```python
from build123d import *

# Parameters (mm, degrees)
CROQUIS1_W                   = 150
CROQUIS1_H                   = 150
SALIENTE_EXTRUIR1_DEPTH      = 10
CROQUIS2_R                   = 67
SALIENTE_EXTRUIR2_DEPTH      = 10
REDONDEO1_R                  = 10
REDONDEO2_R                  = 2
CROQUIS3_R                   = 21
CORTAR_EXTRUIR1_DEPTH        = 108.935165725
TALADRO_DE_MARGEN_PARA_M81_D = 9
TALADRO_DE_MARGEN_PARA_M82_D = 9


with BuildPart() as part:
    # Croquis1 → Saliente-Extruir1 (new body)
    with BuildSketch(Plane(origin=(0, 0, 0), x_dir=(0, 0, -1), z_dir=(1, 0, 0))):
        Rectangle(CROQUIS1_W, CROQUIS1_H)
    extrude(amount=SALIENTE_EXTRUIR1_DEPTH)

    # Croquis2 → Saliente-Extruir2 (add)
    with BuildSketch(Plane(origin=(10, 0, 0), x_dir=(0, 0, -1), z_dir=(1, 0, 0))):
        Circle(CROQUIS2_R)
    extrude(amount=SALIENTE_EXTRUIR2_DEPTH)

    # Redondeo1
    redondeo1_edges = [part.edges().sort_by_distance(p)[0] for p in [
        (5, -75, -75),
        (5, -75, 75),
        (5, 75, 75),
        (5, 75, -75),
    ]]
    fillet(redondeo1_edges, radius=REDONDEO1_R)

    # Redondeo2
    redondeo2_edges = [part.edges().sort_by_distance(p)[0] for p in [
        (10, 0, 67),
    ]]
    fillet(redondeo2_edges, radius=REDONDEO2_R)

    # Croquis3 → Cortar-Extruir1 (cut, through all)
    with BuildSketch(Plane(origin=(20, 0, 0), x_dir=(0, 0, -1), z_dir=(1, 0, 0))):
        Circle(CROQUIS3_R)
    extrude(amount=-CORTAR_EXTRUIR1_DEPTH, mode=Mode.SUBTRACT)

    # Taladro de margen para M81 (through all)
    with Locations(Plane(origin=(10, -7.41730184, 252.760845032), x_dir=(0, 0, -1), z_dir=(1, 0, 0))):
        with Locations((195.760845032, 64.41730184), (309.760845032, 64.41730184)):
            Hole(TALADRO_DE_MARGEN_PARA_M81_D / 2)

    # Taladro de margen para M82 (through all)
    with Locations(Plane(origin=(10, -7.41730184, 252.760845032), x_dir=(0, 0, -1), z_dir=(1, 0, 0))):
        with Locations((309.760845032, -49.58269816), (195.760845032, -49.58269816)):
            Hole(TALADRO_DE_MARGEN_PARA_M82_D / 2)


solid = part.part
```
The model under review builds one solid part; all positions refer to its coordinate system, in mm. A direction names the side the tool comes from. Round coordinates to 2 decimals unless told otherwise and drop trailing zeros. Write each loop counter-clockwise with the first axis right and the second up, starting at its lowest first coordinate (ties: lowest second). Pieces come first, ordered by that corner, then holes. Notation, with made-up numbers: (71, -40) - (75, -40) arc R24 ccw to (75, -14) - close; hole circle Ø7 at (28.5, 43). An arc over 180 degrees is marked (long way). Use one line per item in the form item = value.
Q1. For line 1 (Y direction, x = 6.75, z = 57); line 2 (Y direction, x = 19, z = 0.5); line 3 (X direction, y = 57.5, z = -43), list the stretches that pass through material, from the lowest coordinate up. Write a range as [from, to].
Answer key:
line_1 = [-75, -61.5], [-52.5, 52.5], [61.5, 75]
line_2 = [-67, -20.99], [20.99, 67]
line_3 = [0, 10]
Q2. Tool access review of faces 4 (the flat face through (10, 61, 34)), 5 (the cylindrical face through (10.14, 6.31, -20.03)): name each direction out of +Z, -Z, +X, -X, +Y, -Y from which nothing blocks a thin tool from reaching the whole face with its end or side.
Answer key:
face_4 = +X
face_5 = +X, -X
Q3. Consider section D-D (y = -57). State how many separate pieces and enclosed holes the cut face has, and give its area (3 significant figures).
Answer key:
separate_pieces = 3
enclosed_holes = 0
area = 2,030 mm2
Q4. Consider section C-C (x = 4.25). State the section outline as (y, z) points, and give its area (3 significant figures).
Answer key:
outline = (-75, -65) arc R10 ccw to (-65, -75) - (65, -75) arc R10 ccw to (75, -65) - (75, 65) arc R10 ccw to (65, 75) - (-65, 75) arc R10 ccw to (-75, 65) - close; hole circle Ø9 at (-57, -57); hole circle Ø9 at (-57, 57); hole circle Ø42 at (0, 0); hole circle Ø9 at (57, -57); hole circle Ø9 at (57, 57)
area = 20,800 mm2
Q5. Consider section A-A (y = 0). State the section outline as (x, z) points.
Answer key:
outline = (0, -75) - (10, -75) - (10, -69) arc R2 cw to (12, -67) - (20, -67) - (20, -21) - (0, -21) - close; (0, 21) - (20, 21) - (20, 67) - (12, 67) arc R2 cw to (10, 69) - (10, 75) - (0, 75) - close
Q6. Draft analysis for pull direction Y (two halves, no side actions). For faces 1 (the flat face through (5, -75, 1)), 2 (the cylindrical face through (4.93, 53.01, 59.08)), 3 (the flat face through (0, 18, -16)), state which applies: +Y half, -Y half, draft (parallel to the pull), parting line (faces both ways), or undercut.
Answer key:
face_1 = -Y half
face_2 = undercut
face_3 = draft
Q7. Insertion check: pin 1 Ø1 at (x, z) = (13.5, -7.5) entering from +Y; pin 2 Ø8 at (x, y) = (17, 43) entering from -Z; pin 3 Ø10.5 at (y, z) = (-57, 57) entering from +X. Each pin has a flat end and moves straight along its axis. Give the tip position at first contact, or say it passes through.
Answer key:
pin_1 = 66.63
pin_2 = -54.48
pin_3 = 10
